from build123d import *

# Parameters (mm, degrees)
BOSS_EXTRUDE1_DEPTH      = 0.508
BOSS_EXTRUDE1_DEPTH_BACK = 0.508
SKETCH3_R                = 8.73125
SKETCH3_R_2              = 3.302
FILLET1_R                = 0.13208
FILLET2_R                = 0.174625


with BuildPart() as part:
    # Sketch3 → Boss-Extrude1 (new, two sides: drawn at the far end of the back side and taken through both)
    with BuildSketch(Plane.XY.offset(-BOSS_EXTRUDE1_DEPTH_BACK)):
        Circle(SKETCH3_R)
        Circle(SKETCH3_R_2, mode=Mode.SUBTRACT)
    extrude(amount=BOSS_EXTRUDE1_DEPTH + BOSS_EXTRUDE1_DEPTH_BACK)

    # Fillet1
    fillet1_edges = [part.edges().sort_by_distance(p)[0] for p in [
        (-3.302, 0, 0.508),
        (-3.302, 0, -0.508),
    ]]
    fillet(fillet1_edges, radius=FILLET1_R)

    # Fillet2
    fillet2_edges = [part.edges().sort_by_distance(p)[0] for p in [
        (-8.73125, 0, 0.508),
        (-8.73125, 0, -0.508),
    ]]
    fillet(fillet2_edges, radius=FILLET2_R)


solid = part.part
The listing builds one solid part. Answer for the finished solid, in the listing's coordinates (mm). Coordinates: 2 decimals unless noted, no trailing zeros. Write each loop counter-clockwise with the first axis right and the second up, starting at its lowest first coordinate (ties: lowest second). Pieces come first, ordered by that corner, then holes. Notation, with made-up numbers: (-40, -34) - (2, -34) arc R22 ccw to (2, -10) - close; hole circle Ø11 at (21, 22.5). An arc over 180 degrees is marked (long way). Answer as CSV lines item,"result".
1. Straight lines are drawn through the part: line 1 (Y direction, x = 0, z = -0.05); line 2 (Y direction, x = 3, z = 0.1); line 3 (X direction, y = -1.75, z = -0.4). For each, find the intervals that lie inside material, in ascending order. Write a range as [from, to].
Computed values:
line 1,"y = [-8.73, -3.3], [3.3, 8.73]"
line 2,"y = [-8.2, -1.38], [1.38, 8.2]"
line 3,"x = [-8.54, -2.8], [2.8, 8.54]"
2. Determine the mould class of faces 1 (the flat face through (4, 0, 0.508)), 2 (the cylindrical face through (-6.93, -5.31, 0)), 3 (the cylindrical face through (3.05, -1.26, -0.01)) for opening direction Y: +Y half, -Y half, draft (parallel to the pull), parting line (faces both ways), or undercut.
Computed values:
face 1,"draft"
face 2,"parting line"
face 3,"undercut"
3. Find section C-C (z = 0.1). Give the vertices of the cut face in (x, y).
Computed values:
outline,"circle Ø17.46 at (0, 0); hole circle Ø6.6 at (0, 0)"
4. Find section A-A (y = 0). Give the vertices of the cut face in (x, z), plus the area to 3 significant figures.
Computed values:
outline,"(-8.73, -0.33) arc R0.17 ccw to (-8.56, -0.51) - (-3.43, -0.51) arc R0.13 ccw to (-3.3, -0.38) - (-3.3, 0.38) arc R0.13 ccw to (-3.43, 0.51) - (-8.56, 0.51) arc R0.17 ccw to (-8.73, 0.33) - close; (3.3, -0.38) arc R0.13 ccw to (3.43, -0.51) - (8.56, -0.51) arc R0.17 ccw to (8.73, -0.33) - (8.73, 0.33) arc R0.17 ccw to (8.56, 0.51) - (3.43, 0.51) arc R0.13 ccw to (3.3, 0.38) - close"
area,"11.0 mm²"
